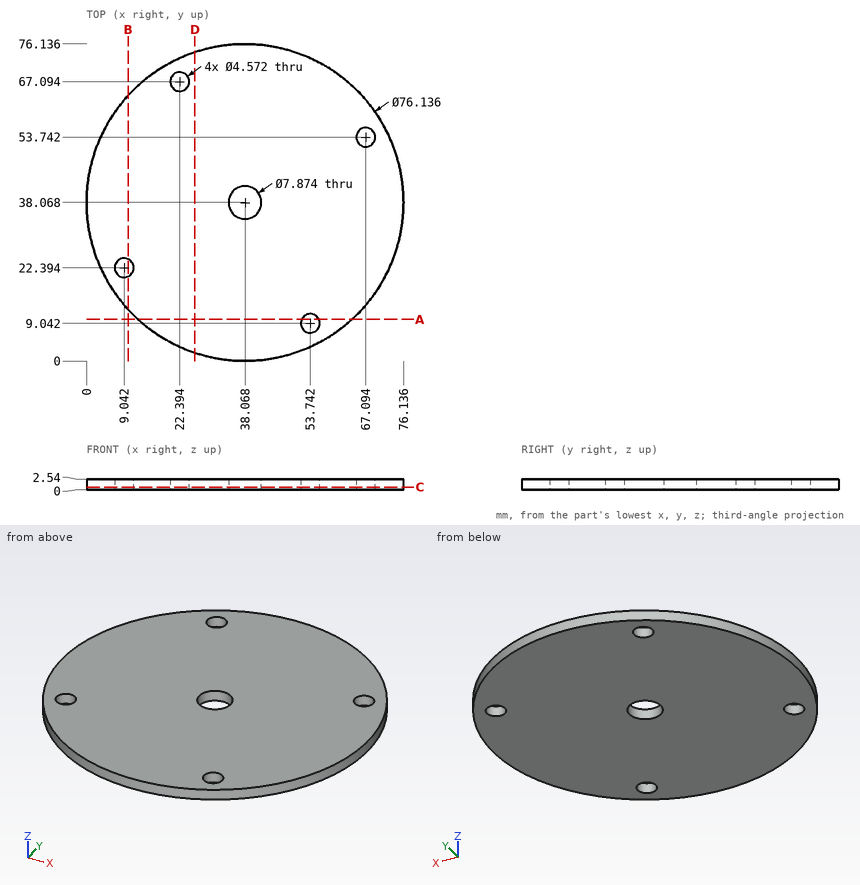
For this review, use the dimensioned drawing (mm, ordinates from the lowest corner) and the shaded views. Coordinates: 2 decimals unless noted, no trailing zeros. Loops run counter-clockwise (first coordinate to the right, second up) from the corner with the lowest first, then second, coordinate; pieces in that order, holes last. Notation, with made-up numbers: (58, 41) -> (90, 41) arc R29 cw to (90, 67) -> close; hole circle Ø10 at (43, 3.25). An arc over 180 degrees is marked (long way). Write each question's results on one line, items separated by ' | '.
Q1. Add section C-C, the plane z = 0.6. State the section outline as (x, y) points (1 decimal).
Taken from the geometry:
outline: circle Ø76.1 at (38.1, 38.1); hole circle Ø4.6 at (9, 22.4); hole circle Ø4.6 at (22.4, 67.1); hole circle Ø7.9 at (38.1, 38.1); hole circle Ø4.6 at (53.7, 9); hole circle Ø4.6 at (67.1, 53.7)
Q2. For pin 1 Ø1 at (y, z) = (36.5, 0.5) entering from -X (3 decimals); pin 2 Ø1 at (x, z) = (53.5, 2) entering from +Y (1 decimal); pin 3 Ø1.5 at (y, z) = (53.5, 1) entering from -X (1 decimal), all flat-tipped, find the tip position at first contact; note any pin that passes through.
Taken from the geometry:
pin 1: x = 0.015 | pin 2: y = 73.1 | pin 3: x = 2.9
Q3. Add section B-B, the plane x = 10. State the section outline as (y, z) points (1 decimal).
Taken from the geometry:
outline: (12.4, 0) -> (20.3, 0) -> (20.3, 2.5) -> (12.4, 2.5) -> close; (24.5, 0) -> (63.8, 0) -> (63.8, 2.5) -> (24.5, 2.5) -> close
Q4. To check wall thickness, follow line 1 along Y through (x, z) = (22, 1.55) (1 decimal); line 2 along X through (y, z) = (67.5, 1.85) (1 decimal); line 3 along Y through (x, z) = (7, 1.2) (1 decimal). State the ranges of each line that lie inside material, in increasing order. Write a range as [from, to].
Taken from the geometry:
line 1: [3.6, 64.8], [69.3, 72.6] | line 2: [13.9, 20.1], [24.6, 62.2] | line 3: [16.1, 21.4], [23.4, 60.1]
Q5. Add section D-D, the plane x = 26. State the section outline as (y, z) points.
Taken from the geometry:
outline: (1.96, 0) -> (74.17, 0) -> (74.17, 2.54) -> (1.96, 2.54) -> close
Q6. Add section A-A, the plane y = 10. State the section outline as (x, z) points (1 decimal), then the cut area to 3 significant figures.
Taken from the geometry:
outline: (12.4, 0) -> (51.7, 0) -> (51.7, 2.5) -> (12.4, 2.5) -> close; (55.8, 0) -> (63.8, 0) -> (63.8, 2.5) -> (55.8, 2.5) -> close | area: 120 mm²
